```python
from build123d import *

# Parameters (mm, degrees)
SKETCH_1_W                       = 2220
SKETCH_1_H                       = 300
EXTRUDE_1_DEPTH                  = 120
SKETCH_2_W                       = 1780
SKETCH_2_H                       = 50
CUT_EXTRUDE_1_DEPTH              = 2244.390291501
SKETCH_3_W                       = 220
SKETCH_3_H                       = 300
EXTRUDE_2_DEPTH                  = 8
SKETCH_4_W                       = 2220
SKETCH_4_H                       = 120
CUT_EXTRUDE_2_DEPTH              = 5
SKETCH_5_W                       = 2220
SKETCH_5_H                       = 120
CUT_EXTRUDE_3_DEPTH              = 5
CUT_EXTRUDE_11_DEPTH             = 2244.832435812
SKETCH_14_W                      = 6
SKETCH_14_H                      = 104
EXTRUDE_3_DEPTH                  = 60
SKETCH_16_W                      = 6
SKETCH_16_H                      = 104
EXTRUDE_4_DEPTH                  = 60
CUT_EXTRUDE_12_DEPTH             = 2139.025490961
PATTERN_LINEAR_2_COUNT           = 2
PATTERN_LINEAR_2_PITCH           = 2000
FILLET_3_R                       = 50
SKETCH_17_W                      = 104
SKETCH_17_H                      = 158
CUT_EXTRUDE_13_DEPTH             = 50
SKETCH_18_W                      = 104
SKETCH_18_H                      = 158
CUT_EXTRUDE_14_DEPTH             = 50
SKETCH_19_R                      = 100
EXTRUDE_5_DEPTH                  = 8
SKETCH_20_R                      = 40
CUT_EXTRUDE_15_DEPTH             = 2245.303009845
SKETCH_21_R                      = 11.5
CUT_EXTRUDE_16_DEPTH             = 2245.303009845
PATTERN_LINEAR_3_COUNT           = 2
PATTERN_LINEAR_3_PITCH           = 80
PATTERN_LINEAR_3_COUNT_DIR2      = 2
PATTERN_LINEAR_3_PITCH_DIR2      = 230
PATTERN_LINEAR_4_COUNT           = 2
PATTERN_LINEAR_4_PITCH           = 2000
PATTERN_LINEAR_4_COPY_1_SKETCH_R = 11.5
PATTERN_LINEAR_4_COPY_1_DEPTH    = 2245.303009845
PATTERN_LINEAR_4_COPY_2_SKETCH_R = 11.5
PATTERN_LINEAR_4_COPY_2_DEPTH    = 2245.303009845
PATTERN_LINEAR_4_COPY_3_SKETCH_R = 11.5
PATTERN_LINEAR_4_COPY_3_DEPTH    = 2245.303009845
SKETCH_22_R                      = 5
CUT_EXTRUDE_17_DEPTH             = 100
PATTERN_LINEAR_5_COUNT           = 2
PATTERN_LINEAR_5_PITCH           = 80
PATTERN_LINEAR_5_COUNT_DIR2      = 2
PATTERN_LINEAR_5_PITCH_DIR2      = 80
PATTERN_LINEAR_6_COUNT           = 2
PATTERN_LINEAR_6_PITCH           = 2000
PATTERN_LINEAR_6_COPY_1_SKETCH_R = 5
PATTERN_LINEAR_6_COPY_1_DEPTH    = 100
PATTERN_LINEAR_6_COPY_2_SKETCH_R = 5
PATTERN_LINEAR_6_COPY_2_DEPTH    = 100
PATTERN_LINEAR_6_COPY_3_SKETCH_R = 5
PATTERN_LINEAR_6_COPY_3_DEPTH    = 100


with BuildPart() as part:
    # 草图1 → 凸台-拉伸1 (new body)
    with BuildSketch(Plane.XY):
        with Locations((1110, 150)):
            Rectangle(SKETCH_1_W, SKETCH_1_H)
    extrude(amount=EXTRUDE_1_DEPTH)

    # 草图2 → 切除-拉伸1 (cut, through all)
    with BuildSketch(Plane.XY.offset(120)):
        with Locations((1110, 275)):
            Rectangle(SKETCH_2_W, SKETCH_2_H)
        with Locations((1110, 25)):
            Rectangle(SKETCH_2_W, SKETCH_2_H)
    extrude(amount=-CUT_EXTRUDE_1_DEPTH, mode=Mode.SUBTRACT)

    # 草图3 → 凸台-拉伸2 (add)
    with BuildSketch(Plane.XY.offset(120)):
        with Locations((110, 150)):
            Rectangle(SKETCH_3_W, SKETCH_3_H)
        with Locations((2110, 150)):
            Rectangle(SKETCH_3_W, SKETCH_3_H)
    extrude(amount=EXTRUDE_2_DEPTH)

    # 草图4 → 切除-拉伸2 (cut)
    with BuildSketch(Plane(origin=(0, 300, 0), x_dir=(1, 0, 0), z_dir=(0, 1, 0))):
        with Locations((1110, -60)):
            Rectangle(SKETCH_4_W, SKETCH_4_H)
    extrude(amount=-CUT_EXTRUDE_2_DEPTH, mode=Mode.SUBTRACT)

    # 草图5 → 切除-拉伸3 (cut)
    with BuildSketch(Plane.XZ):
        with Locations((1110, 60)):
            Rectangle(SKETCH_5_W, SKETCH_5_H)
    extrude(amount=-CUT_EXTRUDE_3_DEPTH, mode=Mode.SUBTRACT)

    # 草图13 → 切除-拉伸11 (cut, through all)
    with BuildSketch(Plane(origin=(2220, 0, 0), x_dir=(0, 0, -1), z_dir=(1, 0, 0))):
        Polygon((-112, 235), (-8, 235), (-8, 250), (0, 250), (0, 295), (-112, 295), align=None)
        Polygon((-112, 5), (0, 5), (0, 50), (-8, 50), (-8, 65), (-112, 65), align=None)
    extrude(amount=-CUT_EXTRUDE_11_DEPTH, mode=Mode.SUBTRACT)

    # 草图14 → 凸台-拉伸3 (add)
    with BuildSketch(Plane(origin=(0, 235, 0), x_dir=(1, 0, 0), z_dir=(0, 1, 0))):
        with Locations((2110, -60)):
            Rectangle(SKETCH_14_W, SKETCH_14_H)
    extrude_3 = extrude(amount=EXTRUDE_3_DEPTH)

    # 草图16 → 凸台-拉伸4 (add)
    with BuildSketch(Plane.XZ.offset(-65)):
        with Locations((2110, 60)):
            Rectangle(SKETCH_16_W, SKETCH_16_H)
    extrude_4 = extrude(amount=EXTRUDE_4_DEPTH)

    # 草图15 → 切除-拉伸12 (cut, through all)
    with BuildSketch(Plane(origin=(2113, 0, 0), x_dir=(0, 0, -1), z_dir=(1, 0, 0))):
        Polygon((-8, 295), (-8, 250), (-112, 295), align=None)
        Polygon((-8, 50), (-112, 5), (-8, 5), align=None)
    cut_extrude_12 = extrude(amount=-CUT_EXTRUDE_12_DEPTH, mode=Mode.SUBTRACT)

    # 阵列(线性)2: 凸台-拉伸3, 凸台-拉伸4, 切除-拉伸12 ×2
    with Locations(*[(-i * PATTERN_LINEAR_2_PITCH, 0, 0) for i in range(1, PATTERN_LINEAR_2_COUNT)]):
        add(extrude_3)
        add(extrude_4)
        add(cut_extrude_12, mode=Mode.SUBTRACT)

    # 圆角3
    # the kernel refuses this fillet: 50 mm, written as the material it adds along each edge
    with BuildSketch(Plane(origin=(220, 250, 120), x_dir=(0, 1, 0), z_dir=(0, 0, -1))) as fillet_3_piece_1_section:
        with BuildLine():
            CenterArc((FILLET_3_R, FILLET_3_R), FILLET_3_R, 180, 90)
            Line((0, FILLET_3_R), (0, 0))
            Line((0, 0), (FILLET_3_R, 0))
        make_face()
    fillet_3_piece_1 = extrude(amount=8, mode=Mode.PRIVATE)
    fillet_3_piece_1 = split(fillet_3_piece_1, bisect_by=Plane(origin=(231.177032, 295, 116), z_dir=(0, -1, 0)), keep=Keep.TOP, mode=Mode.PRIVATE)
    add(fillet_3_piece_1)
    with BuildSketch(Plane(origin=(2000, 250, 120), x_dir=(-1, 0, 0), z_dir=(0, 0, -1))) as fillet_3_piece_2_section:
        with BuildLine():
            CenterArc((FILLET_3_R, FILLET_3_R), FILLET_3_R, 180, 90)
            Line((0, FILLET_3_R), (0, 0))
            Line((0, 0), (FILLET_3_R, 0))
        make_face()
    fillet_3_piece_2 = extrude(amount=8, mode=Mode.PRIVATE)
    fillet_3_piece_2 = split(fillet_3_piece_2, bisect_by=Plane(origin=(1988.822968, 295, 116), z_dir=(0, -1, 0)), keep=Keep.TOP, mode=Mode.PRIVATE)
    add(fillet_3_piece_2)
    with BuildSketch(Plane(origin=(2000, 50, 120), x_dir=(-1, 0, 0), z_dir=(0, 0, -1))) as fillet_3_piece_3_section:
        with BuildLine():
            CenterArc((FILLET_3_R, -FILLET_3_R), FILLET_3_R, 90, 90)
            Line((0, -FILLET_3_R), (0, 0))
            Line((0, 0), (FILLET_3_R, 0))
        make_face()
    fillet_3_piece_3 = extrude(amount=8, mode=Mode.PRIVATE)
    fillet_3_piece_3 = split(fillet_3_piece_3, bisect_by=Plane(origin=(1988.822968, 5, 116), z_dir=(0, 1, 0)), keep=Keep.TOP, mode=Mode.PRIVATE)
    add(fillet_3_piece_3)
    with BuildSketch(Plane(origin=(220, 50, 120), x_dir=(0, -1, 0), z_dir=(0, 0, -1))) as fillet_3_piece_4_section:
        with BuildLine():
            CenterArc((FILLET_3_R, -FILLET_3_R), FILLET_3_R, 90, 90)
            Line((0, -FILLET_3_R), (0, 0))
            Line((0, 0), (FILLET_3_R, 0))
        make_face()
    fillet_3_piece_4 = extrude(amount=8, mode=Mode.PRIVATE)
    fillet_3_piece_4 = split(fillet_3_piece_4, bisect_by=Plane(origin=(231.177032, 5, 116), z_dir=(0, 1, 0)), keep=Keep.TOP, mode=Mode.PRIVATE)
    add(fillet_3_piece_4)

    # 草图17 → 切除-拉伸13 (cut)
    with BuildSketch(Plane.ZY):
        with Locations((60, 150)):
            Rectangle(SKETCH_17_W, SKETCH_17_H)
    extrude(amount=-CUT_EXTRUDE_13_DEPTH, mode=Mode.SUBTRACT)

    # 草图18 → 切除-拉伸14 (cut)
    with BuildSketch(Plane(origin=(2220, 0, 0), x_dir=(0, 0, -1), z_dir=(1, 0, 0))):
        with Locations((-60, 150)):
            Rectangle(SKETCH_18_W, SKETCH_18_H)
    extrude(amount=-CUT_EXTRUDE_14_DEPTH, mode=Mode.SUBTRACT)

    # 草图19 → 凸台-拉伸5 (add)
    with BuildSketch(Plane(origin=(0, 0, 0), x_dir=(-1, 0, 0), z_dir=(0, 0, -1))):
        with Locations(Location((-1110, 150, 0), (0, 0, 270))):
            Circle(SKETCH_19_R)
    extrude(amount=EXTRUDE_5_DEPTH)

    # 草图20 → 切除-拉伸15 (cut, through all)
    with BuildSketch(Plane(origin=(0, 0, -8), x_dir=(-1, 0, 0), z_dir=(0, 0, -1))):
        with Locations((-1110, 150)):
            Circle(SKETCH_20_R)
    extrude(amount=-CUT_EXTRUDE_15_DEPTH, mode=Mode.SUBTRACT)

    # 草图21 → 切除-拉伸16 (cut, through all)
    with BuildSketch(Plane.XY.offset(128)):
        with Locations((2150, 35)):
            Circle(SKETCH_21_R)
    cut_extrude_16 = extrude(amount=-CUT_EXTRUDE_16_DEPTH, mode=Mode.SUBTRACT)

    # 阵列(线性)3: Cut-Extrude 16 2 × 2
    with Locations(*[(-i * PATTERN_LINEAR_3_PITCH, j * PATTERN_LINEAR_3_PITCH_DIR2, 0) for i in range(PATTERN_LINEAR_3_COUNT) for j in range(PATTERN_LINEAR_3_COUNT_DIR2) if (i, j) != (0, 0)]):
        add(cut_extrude_16, mode=Mode.SUBTRACT)

    # 阵列(线性)4: 切除-拉伸16 ×2
    with Locations(*[(-i * PATTERN_LINEAR_4_PITCH, 0, 0) for i in range(1, PATTERN_LINEAR_4_COUNT)]):
        add(cut_extrude_16, mode=Mode.SUBTRACT)

    # 阵列(线性)4 copy 1 sketch → 阵列(线性)4 copy 1 (cut, through all)
    with BuildSketch(Plane(origin=(-2000, 230, 128), x_dir=(1, 0, 0), z_dir=(0, 0, 1))):
        with Locations((2150, 35)):
            Circle(PATTERN_LINEAR_4_COPY_1_SKETCH_R)
    extrude(amount=-PATTERN_LINEAR_4_COPY_1_DEPTH, mode=Mode.SUBTRACT)

    # 阵列(线性)4 copy 2 sketch → 阵列(线性)4 copy 2 (cut, through all)
    with BuildSketch(Plane(origin=(-2080, 0, 128), x_dir=(1, 0, 0), z_dir=(0, 0, 1))):
        with Locations((2150, 35)):
            Circle(PATTERN_LINEAR_4_COPY_2_SKETCH_R)
    extrude(amount=-PATTERN_LINEAR_4_COPY_2_DEPTH, mode=Mode.SUBTRACT)

    # 阵列(线性)4 copy 3 sketch → 阵列(线性)4 copy 3 (cut, through all)
    with BuildSketch(Plane(origin=(-2080, 230, 128), x_dir=(1, 0, 0), z_dir=(0, 0, 1))):
        with Locations((2150, 35)):
            Circle(PATTERN_LINEAR_4_COPY_3_SKETCH_R)
    extrude(amount=-PATTERN_LINEAR_4_COPY_3_DEPTH, mode=Mode.SUBTRACT)

    # 草图22 → 切除-拉伸17 (cut)
    with BuildSketch(Plane(origin=(0, 0, 0), x_dir=(-1, 0, 0), z_dir=(0, 0, -1))):
        with Locations((-2150, 190)):
            Circle(SKETCH_22_R)
    cut_extrude_17 = extrude(amount=-CUT_EXTRUDE_17_DEPTH, mode=Mode.SUBTRACT)

    # 阵列(线性)5: Cut-Extrude 17 2 × 2
    with Locations(*[(-i * PATTERN_LINEAR_5_PITCH, -j * PATTERN_LINEAR_5_PITCH_DIR2, 0) for i in range(PATTERN_LINEAR_5_COUNT) for j in range(PATTERN_LINEAR_5_COUNT_DIR2) if (i, j) != (0, 0)]):
        add(cut_extrude_17, mode=Mode.SUBTRACT)

    # 阵列(线性)6: 切除-拉伸17 ×2
    with Locations(*[(-i * PATTERN_LINEAR_6_PITCH, 0, 0) for i in range(1, PATTERN_LINEAR_6_COUNT)]):
        add(cut_extrude_17, mode=Mode.SUBTRACT)

    # 阵列(线性)6 copy 1 sketch → 阵列(线性)6 copy 1 (cut)
    with BuildSketch(Plane(origin=(-2000, -80, 0), x_dir=(-1, 0, 0), z_dir=(0, 0, -1))):
        with Locations((-2150, 190)):
            Circle(PATTERN_LINEAR_6_COPY_1_SKETCH_R)
    extrude(amount=-PATTERN_LINEAR_6_COPY_1_DEPTH, mode=Mode.SUBTRACT)

    # 阵列(线性)6 copy 2 sketch → 阵列(线性)6 copy 2 (cut)
    with BuildSketch(Plane(origin=(-2080, 0, 0), x_dir=(-1, 0, 0), z_dir=(0, 0, -1))):
        with Locations((-2150, 190)):
            Circle(PATTERN_LINEAR_6_COPY_2_SKETCH_R)
    extrude(amount=-PATTERN_LINEAR_6_COPY_2_DEPTH, mode=Mode.SUBTRACT)

    # 阵列(线性)6 copy 3 sketch → 阵列(线性)6 copy 3 (cut)
    with BuildSketch(Plane(origin=(-2080, -80, 0), x_dir=(-1, 0, 0), z_dir=(0, 0, -1))):
        with Locations((-2150, 190)):
            Circle(PATTERN_LINEAR_6_COPY_3_SKETCH_R)
    extrude(amount=-PATTERN_LINEAR_6_COPY_3_DEPTH, mode=Mode.SUBTRACT)


solid = part.part
```
Geometry: final body of the model. Coordinates: model frame, mm. A direction names the side the tool comes from. Round coordinates to 2 decimals unless told otherwise and drop trailing zeros. Order: outer loops, then holes, each group sorted by start corner. A loop starts at its lowest first (then second) coordinate and runs counter-clockwise, first axis right, second up. Notation, with made-up numbers: M -26,-24.75 L 15,-24.75 A25 ccw 15,-9.75 Z; hole C -23,25.25 d3. An arc over 180 degrees is marked long. Use one line per item in the form item = value. Start each with the question number.
Q1. Cut plane B-B (x = 1412). Return loops of the section in (y, z).
Q2. Cut plane C-C (z = 64). Count the separate pieces of the cut face and the enclosed holes in it, and give its area (3 significant figures).
Q3. Mould query, pull axis X, two halves, no side actions, for faces 1 (the face through (1010.85, 163.02, -3.94)), 2 (the face through (1142, 126, 55)), 3 (the face through (25, 71, 59)). Classes: +X half, -X half, draft (parallel to the pull), parting line (faces both ways), or undercut.
Q4. Cut plane A-A (y = 150). Return loops of the section in (x, z).
Q5. Access query for faces 4 (the face through (2167, 265, 112)), 5 (the face through (113, 42, 71)), 6 (the face through (1124, 235, 61)). Directions: +Z, -Z, +X, -X, +Y, -Y. A direction counts if a zero-diameter tool reaches every point of the face in a straight line with its end or side. Return the directions, or none.
Q6. Material intervals for line 1 (Y direction, x = 150, z = 122); line 2 (Y direction, x = 2150, z = 116.75); line 3 (Z direction, x = 1963, y = 237), sorted ascending. Write a range as [from, to].
Q7. Pin query (flat end, axial travel): pin 1 Ø12 at (y, z) = (97, 62.5) entering from -X; pin 2 Ø11.5 at (x, y) = (2150, 190) entering from -Z; pin 3 Ø2 at (x, z) = (1855.5, 111.5) entering from -Y. Return the tip coordinate at first contact, or that it passes through.
Geometry results:
q1.outline = M 50,0 L 250,0 L 250,8 L 235,8 L 235,112 L 250,112 L 250,120 L 50,120 L 50,112 L 65,112 L 65,8 L 50,8 Z
q2.separate_pieces = 1
q2.enclosed_holes = 9
q2.area = 357,000 mm^2
q3.face_1 = parting line
q3.face_2 = undercut
q3.face_3 = draft
q4.outline = M 0,0 L 1010,0 L 1010,-8 L 1070,-8 L 1070,120 L 220,120 L 220,128 L 0,128 L 0,112 L 50,112 L 50,8 L 0,8 Z; M 1150,-8 L 1210,-8 L 1210,0 L 2220,0 L 2220,8 L 2170,8 L 2170,112 L 2220,112 L 2220,128 L 2000,128 L 2000,120 L 1150,120 Z
q5.face_4 = +X, +Y
q5.face_5 = -Y
q5.face_6 = +Y
q6.line_1 = [0, 23.5], [46.5, 253.5], [276.5, 300]
q6.line_2 = [5, 23.5], [46.5, 253.5], [276.5, 295]
q6.line_3 = [0, 8], [112, 120]
q7.pin_1 = 50
q7.pin_2 = 0
q7.pin_3 = 50
